```python
from build123d import *

# Parameters (mm, degrees)
CROQUIS1_R              = 16
SALIENTE_EXTRUIR1_DEPTH = 2
CROQUIS4_R              = 14
SALIENTE_EXTRUIR2_DEPTH = 3
CROQUIS5_R              = 16
SALIENTE_EXTRUIR3_DEPTH = 2
CORTAR_EXTRUIR1_DEPTH   = 24.685438565
CHAFL_N1_SIZE           = 1
CHAFL_N2_SIZE           = 1


with BuildPart() as part:
    # Croquis1 → Saliente-Extruir1 (new body)
    with BuildSketch(Plane(origin=(0, 0, 0), x_dir=(1, 0, 0), z_dir=(0, 1, 0))):
        with Locations(Location((0, 0, 0), (0, 0, 270))):
            Circle(CROQUIS1_R)
    extrude(amount=SALIENTE_EXTRUIR1_DEPTH)

    # Croquis4 → Saliente-Extruir2 (add)
    with BuildSketch(Plane(origin=(0, 2, 0), x_dir=(1, 0, 0), z_dir=(0, 1, 0))):
        with Locations(Location((0, 0, 0), (0, 0, 270))):
            Circle(CROQUIS4_R)
    extrude(amount=SALIENTE_EXTRUIR2_DEPTH)

    # Croquis5 → Saliente-Extruir3 (add)
    with BuildSketch(Plane(origin=(0, 5, 0), x_dir=(1, 0, 0), z_dir=(0, 1, 0))):
        with Locations(Location((0, 0, 0), (0, 0, 270))):
            Circle(CROQUIS5_R)
    extrude(amount=SALIENTE_EXTRUIR3_DEPTH)

    # Croquis6 → Cortar-Extruir1 (cut, through all)
    with BuildSketch(Plane(origin=(0, 7, 0), x_dir=(1, 0, 0), z_dir=(0, 1, 0))):
        with BuildLine():
            Line((-2.645751311, -3), (2.645751311, -3))
            ThreePointArc((2.645751311, -3), (4, 0), (2.645751311, 3))
            Line((2.645751311, 3), (-2.645751311, 3))
            ThreePointArc((-2.645751311, 3), (-4, 0), (-2.645751311, -3))
        make_face()
    extrude(amount=-CORTAR_EXTRUIR1_DEPTH, mode=Mode.SUBTRACT)

    # Chaflán1
    chafl_n1_edges = [part.edges().sort_by_distance(p)[0] for p in [
        (0, 7, -16),
    ]]
    chamfer(chafl_n1_edges, length=CHAFL_N1_SIZE)

    # Chaflán2
    chafl_n2_edges = [part.edges().sort_by_distance(p)[0] for p in [
        (0, 0, -16),
    ]]
    chamfer(chafl_n2_edges, length=CHAFL_N2_SIZE)


solid = part.part
```
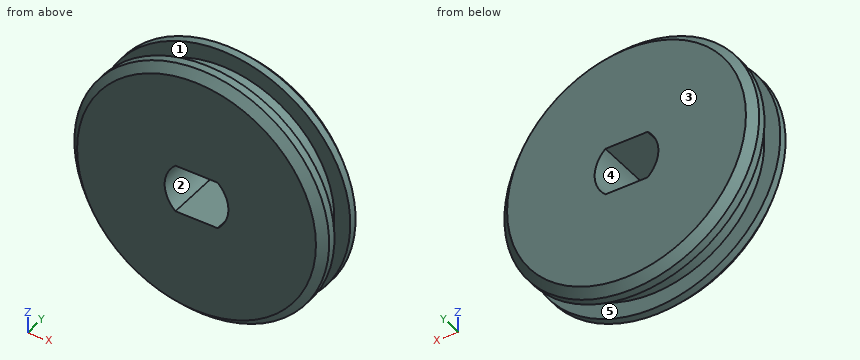
Check sheet for the modelled part. Datum: model origin and axes. Units: mm. Face numbers are marked on the shaded views. A direction names the side the tool comes from. Give positions to 0.01 mm unless a question says otherwise; leave off trailing zeros. Loops run counter-clockwise (first coordinate to the right, second up) from the corner with the lowest first, then second, coordinate; pieces in that order, holes last. Notation, with made-up numbers: M -39,36.5 L -29,36.5 A30 ccw -29,69.5 Z; hole C 84.25,35.25 d1. An arc over 180 degrees is marked long. Answer as CSV lines item,"result".
Item 1: Scan lines: L1, parallel to Z at x = -0.5, y = 2.5; L2, parallel to Y at x = 13, z = 8.5; L3, parallel to X at y = 3.25, z = 1. Record each from-to range of solid material in increasing order.
Reply:
L1,"-13.99 to -3, 3 to 13.99"
L2,"0.53 to 2, 5 to 6.47"
L3,"-13.96 to -3.87, 3.87 to 13.96"
Item 2: Sectioned sample at D-D, the plane y = 1.5. Enter the section's corners in (x, z), then the cut area to 3 significant figures.
Reply:
outline,"C 0,0 d32; hole M -2.65,-3 L 2.65,-3 A4 ccw 2.65,3 L -2.65,3 A4 ccw Z"
area,"761 mm^2"
Item 3: Depth check by flat-ended pin: pin 1 Ø3 at (y, z) = (1.5, -4.5) entering from -X; pin 2 Ø2 at (y, z) = (5, 11.5) entering from +X; pin 3 Ø2 at (y, z) = (2.5, -9.5) entering from +X. Enter the tip coordinate at first touch or a pass-through.
Reply:
pin 1,"x = -15.72"
pin 2,"x = 12.07"
pin 3,"x = 13.47"
Item 4: Sectioned sample at B-B, the plane z = 0. Enter the section's corners in (x, y).
Reply:
outline,"M -16,1 L -15,0 L -4,0 L -4,7 L -15,7 L -16,6 L -16,5 L -14,5 L -14,2 L -16,2 Z; M 4,0 L 15,0 L 16,1 L 16,2 L 14,2 L 14,5 L 16,5 L 16,6 L 15,7 L 4,7 Z"
Item 5: Sectioned sample at C-C, the plane y = 4.25. Enter the section's corners in (x, z).
Reply:
outline,"C 0,0 d28; hole M -2.65,-3 L 2.65,-3 A4 ccw 2.65,3 L -2.65,3 A4 ccw Z"
Item 6: Set-up check for the marked faces 1, 2 and 3: record each of +Z, -Z, +X, -X, +Y, -Y from which the full face is reachable in a straight line by a thin tool's end or side.
Reply:
face 1,"none"
face 2,"+Y, -Y"
face 3,"+Z, -Z, +X, -X, +Y"
Item 7: Sectioned sample at A-A, the plane x = 0. Enter the section's corners in (y, z).
Reply:
outline,"M 0,-15 L 1,-16 L 2,-16 L 2,-14 L 5,-14 L 5,-16 L 6,-16 L 7,-15 L 7,-3 L 0,-3 Z; M 0,3 L 7,3 L 7,15 L 6,16 L 5,16 L 5,14 L 2,14 L 2,16 L 1,16 L 0,15 Z"
Item 8: Draft check along X on the marked faces 4 and 5. Enter one of: pulls with the +X half, pulls with the -X half, needs draft (parallel to the pull), parting line crosses it, or undercut.
Reply:
face 4,"undercut"
face 5,"needs draft"
